Source: three-view drawing plus pictorial views. Frame: mm from the lowest corner of the part. Give positions to 0.01 mm unless a question says otherwise; leave off trailing zeros. Order: outer loops, then holes, each group sorted by start corner. A loop starts at its lowest first (then second) coordinate and runs counter-clockwise, first axis right, second up. Notation, with made-up numbers: (18, -13.75) -> (52, -13.75) arc R17 ccw to (52, 3.25) -> close; hole circle Ø6 at (-38, 12). An arc over 180 degrees is marked (long way). Answer in a Markdown table with one row per item. Add a question column.
Q1. Contact query for flat-ended pins moving along their axis: P1, Ø1.5, axis at y = 2, z = 21.5, coming from the -X side; P2, Ø1, axis at x = 13, y = 1.5, coming from the +Z side; P3, Ø1.5, axis at y = 1.5, z = 21, coming from the +X side. Output: stop coordinate, or through.
Q2. Cut plane A-A on x = 10. Return the cut outline in (y, z), and give its area (3 significant figures).
Q3. Cut plane D-D on x = 29.5. Return the cut outline in (y, z), and give its area (3 significant figures).
Q4. Cut plane C-C on z = 7. Return the cut outline in (x, y).
Q5. Line query: line 1 along X through (y, z) = (2, 7); line 2 along X through (y, z) = (2.1, 10.25); line 3 along Z through (x, y) = (60, 0.95). Output: solid intervals per line, ascending. Write a range as from..to.
Q6. Cut plane B-B on y = 2.5. Return the cut outline in (x, z).
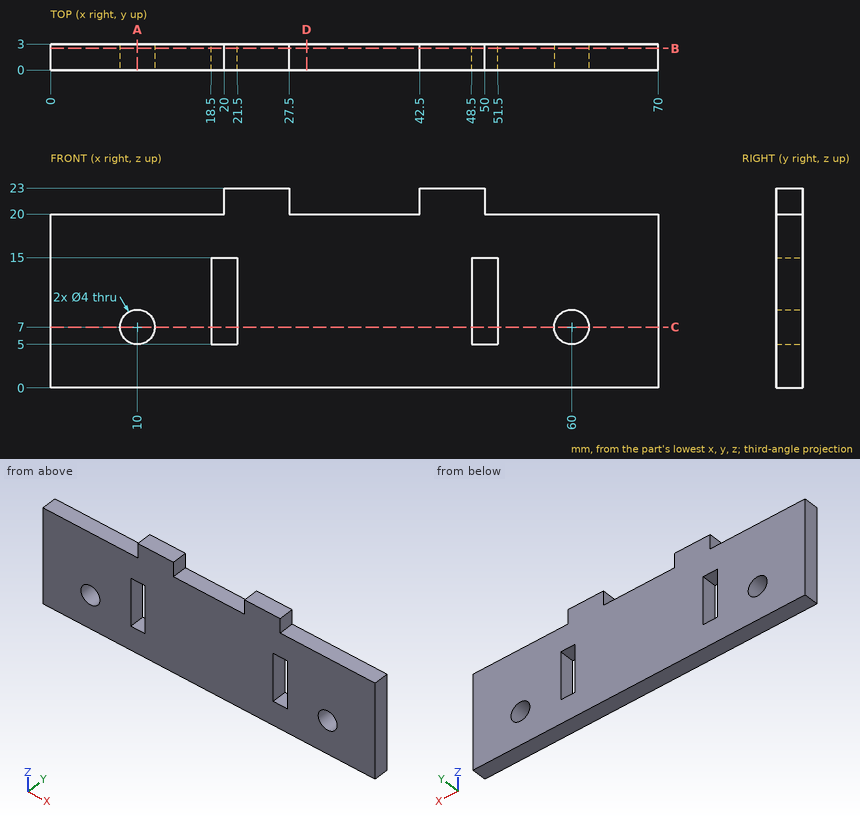
Completed:
| question | item | result |
|---|---|---|
| 1 | P1 | stops at x = 20 |
| 1 | P2 | stops at z = 20 |
| 1 | P3 | stops at x = 50 |
| 2 | outline | (0, 0) -> (3, 0) -> (3, 5) -> (0, 5) -> close; (0, 9) -> (3, 9) -> (3, 20) -> (0, 20) -> close |
| 2 | area | 48.0 mm² |
| 3 | outline | (0, 0) -> (3, 0) -> (3, 20) -> (0, 20) -> close |
| 3 | area | 60.0 mm² |
| 4 | outline | (0, 0) -> (8, 0) -> (8, 3) -> (0, 3) -> close; (12, 0) -> (18.5, 0) -> (18.5, 3) -> (12, 3) -> close; (21.5, 0) -> (48.5, 0) -> (48.5, 3) -> (21.5, 3) -> close; (51.5, 0) -> (58, 0) -> (58, 3) -> (51.5, 3) -> close; (62, 0) -> (70, 0) -> (70, 3) -> (62, 3) -> close |
| 5 | line 1 | x = 0..8, 12..18.5, 21.5..48.5, 51.5..58, 62..70 |
| 5 | line 2 | x = 0..18.5, 21.5..48.5, 51.5..70 |
| 5 | line 3 | z = 0..5, 9..20 |
| 6 | outline | (0, 0) -> (70, 0) -> (70, 20) -> (50, 20) -> (50, 23) -> (42.5, 23) -> (42.5, 20) -> (27.5, 20) -> (27.5, 23) -> (20, 23) -> (20, 20) -> (0, 20) -> close; hole circle Ø4 at (10, 7); hole (18.5, 5) -> (21.5, 5) -> (21.5, 15) -> (18.5, 15) -> close; hole (48.5, 5) -> (51.5, 5) -> (51.5, 15) -> (48.5, 15) -> close; hole circle Ø4 at (60, 7) |
